Input: part model. Units: mm. Frame: model coordinates. A direction names the side the tool comes from. Give positions to 0.01 mm unless a question says otherwise; leave off trailing zeros. Write each loop counter-clockwise with the first axis right and the second up, starting at its lowest first coordinate (ties: lowest second). Pieces come first, ordered by that corner, then holes.
```python
from build123d import *

# Parameters (mm, degrees)
SKETCH1_R            = 2.9
BOSS_EXTRUDE1_DEPTH  = 7.5
SKETCH2_W            = 1
SKETCH2_H            = 1
CUT_EXTRUDE1_DEPTH   = 7.5
SKETCH8_W            = 1.3
SKETCH8_H            = 7.5
BOSS_EXTRUDE4_DEPTH  = 1
CIRPATTERN3_COUNT    = 8
SKETCH10_W           = 1.3
SKETCH10_H           = 3.5
BOSS_EXTRUDE6_DEPTH  = 1
SKETCH11_W           = 1.3
SKETCH11_H           = 3.5
BOSS_EXTRUDE7_DEPTH  = 1
SKETCH12_W           = 1.3
SKETCH12_H           = 3.5
BOSS_EXTRUDE8_DEPTH  = 1
SKETCH14_W           = 1.3
SKETCH14_H           = 3.5
BOSS_EXTRUDE9_DEPTH  = 1
SKETCH15_W           = 1.3
SKETCH15_H           = 3.5
BOSS_EXTRUDE10_DEPTH = 1
SKETCH16_W           = 1.3
SKETCH16_H           = 3.5
BOSS_EXTRUDE11_DEPTH = 1
SKETCH17_W           = 1.3
SKETCH17_H           = 3.43512081
BOSS_EXTRUDE12_DEPTH = 1
SKETCH18_W           = 1.3
SKETCH18_H           = 3.5
BOSS_EXTRUDE13_DEPTH = 1


with BuildPart() as part:
    # Sketch1 → Boss-Extrude1 (new body)
    with BuildSketch(Plane(origin=(0, 0, 0), x_dir=(1, 0, 0), z_dir=(0, 1, 0))):
        Circle(SKETCH1_R)
    extrude(amount=BOSS_EXTRUDE1_DEPTH)

    # Sketch2 → Cut-Extrude1 (cut)
    with BuildSketch(Plane.XZ):
        with BuildLine():
            Line((0.5, 0.5), (0.5, 2.2))
            ThreePointArc((0.5, 2.2), (0, 2.7), (-0.5, 2.2))
            Line((-0.5, 2.2), (-0.5, 0.5))
            Line((-0.5, 0.5), (0.5, 0.5))
        make_face()
        Rectangle(SKETCH2_W, SKETCH2_H)
        with BuildLine():
            Line((0.5, -2.2), (0.5, -0.5))
            Line((0.5, -0.5), (-0.5, -0.5))
            Line((-0.5, -0.5), (-0.5, -2.2))
            ThreePointArc((-0.5, -2.2), (0, -2.7), (0.5, -2.2))
        make_face()
        with BuildLine():
            Line((2.2, 0.5), (0.5, 0.5))
            Line((0.5, 0.5), (0.5, -0.5))
            Line((0.5, -0.5), (2.2, -0.5))
            ThreePointArc((2.2, -0.5), (2.7, 0), (2.2, 0.5))
        make_face()
        with BuildLine():
            Line((-0.5, -0.5), (-0.5, 0.5))
            Line((-0.5, 0.5), (-2.2, 0.5))
            ThreePointArc((-2.2, 0.5), (-2.7, 0), (-2.2, -0.5))
            Line((-2.2, -0.5), (-0.5, -0.5))
        make_face()
    extrude(amount=-CUT_EXTRUDE1_DEPTH, mode=Mode.SUBTRACT)

    # Sketch8 → Boss-Extrude4 (add)
    with BuildSketch(Plane(origin=(2.8, 0, 0), x_dir=(0, 0, -1), z_dir=(1, 0, 0))):
        with Locations((0.006709133, 3.75)):
            Rectangle(SKETCH8_W, SKETCH8_H)
    boss_extrude4 = extrude(amount=BOSS_EXTRUDE4_DEPTH)

    # CirPattern3: Boss-Extrude4 ×8 about axis
    cirpattern3_axis = Axis((0, 0, 0), (0, 1, 0))
    for i in range(1, CIRPATTERN3_COUNT):
        add(boss_extrude4.rotate(cirpattern3_axis, i * 360 / CIRPATTERN3_COUNT))

    # Sketch10 → Boss-Extrude6 (add)
    with BuildSketch(Plane(origin=(0, 0, -3.8), x_dir=(-1, 0, 0), z_dir=(0, 0, -1))):
        with Locations((0.006709133, 3.75)):
            Rectangle(SKETCH10_W, SKETCH10_H)
    extrude(amount=BOSS_EXTRUDE6_DEPTH)

    # Sketch11 → Boss-Extrude7 (add)
    with BuildSketch(Plane(origin=(-2.687005769, 0, -2.687005769), x_dir=(-0.707106781, 0, 0.707106781), z_dir=(-0.707106781, 0, -0.707106781))):
        with Locations((0.006709133, 3.75)):
            Rectangle(SKETCH11_W, SKETCH11_H)
    extrude(amount=BOSS_EXTRUDE7_DEPTH)

    # Sketch12 → Boss-Extrude8 (add)
    with BuildSketch(Plane.ZY.offset(3.8)):
        with Locations((0.006709133, 3.75)):
            Rectangle(SKETCH12_W, SKETCH12_H)
    extrude(amount=BOSS_EXTRUDE8_DEPTH)

    # Sketch14 → Boss-Extrude9 (add)
    with BuildSketch(Plane(origin=(-2.687005769, 0, 2.687005769), x_dir=(0.707106781, 0, 0.707106781), z_dir=(-0.707106781, 0, 0.707106781))):
        with Locations((0.006709133, 3.75)):
            Rectangle(SKETCH14_W, SKETCH14_H)
    extrude(amount=BOSS_EXTRUDE9_DEPTH)

    # Sketch15 → Boss-Extrude10 (add)
    with BuildSketch(Plane.XY.offset(3.8)):
        with Locations((0.006709133, 3.75)):
            Rectangle(SKETCH15_W, SKETCH15_H)
    extrude(amount=BOSS_EXTRUDE10_DEPTH)

    # Sketch16 → Boss-Extrude11 (add)
    with BuildSketch(Plane(origin=(2.687005769, 0, 2.687005769), x_dir=(0.707106781, 0, -0.707106781), z_dir=(0.707106781, 0, 0.707106781))):
        with Locations((0.006709133, 3.75)):
            Rectangle(SKETCH16_W, SKETCH16_H)
    extrude(amount=BOSS_EXTRUDE11_DEPTH)

    # Sketch17 → Boss-Extrude12 (add)
    with BuildSketch(Plane(origin=(3.8, 0, 0), x_dir=(0, 0, -1), z_dir=(1, 0, 0))):
        with Locations((0.006709133, 3.782439595)):
            Rectangle(SKETCH17_W, SKETCH17_H)
    extrude(amount=BOSS_EXTRUDE12_DEPTH)

    # Sketch18 → Boss-Extrude13 (add)
    with BuildSketch(Plane(origin=(2.687005769, 0, -2.687005769), x_dir=(-0.707106781, 0, -0.707106781), z_dir=(0.707106781, 0, -0.707106781))):
        with Locations((0.006709133, 3.75)):
            Rectangle(SKETCH18_W, SKETCH18_H)
    extrude(amount=BOSS_EXTRUDE13_DEPTH)


solid = part.part
```
Q1. Access query for faces 1 (the flat face through (4, 5.5, 0)), 2 (the flat face through (2.99, 3.7, -2.08)), 3 (the flat face through (2.07, 3.7, -3)), 4 (the flat face through (-2.689, 1.014, 2.685)). Directions: +Z, -Z, +X, -X, +Y, -Y. A direction counts if a zero-diameter tool reaches every point of the face in a straight line with its end or side. Return the directions, or none.
Q2. Mould query, pull axis Z, two halves, no side actions, for faces 5 (the flat face through (-0.5, 4, 1)), 6 (the flat face through (0, 4, -4.8)), 7 (the flat face through (3, 2, 3)), 8 (the flat face through (-2.99, 3.7, 2.08)). Classes: +Z half, -Z half, draft (parallel to the pull), parting line (faces both ways), or undercut.
Q3. Pin query (flat end, axial travel): pin 1 (0.6 mm diameter, centred on y = 4.5, z = -4, fed in from -X); pin 2 (0.8 mm diameter, centred on x = -1.5, y = 2, fed in from -Z); pin 3 (2 mm diameter, centred on x = 3.5, y = 3, fed in from +Z). Return the tip coordinate at first contact, or that it passes through.
Q4. Material intervals for line 1 along X through (y, z) = (4.75, 0); line 2 along Z through (x, y) = (0, 6.25); line 3 along X through (y, z) = (2.25, 3.25), sorted ascending.
Q5. Section A-A, the plane x = 0. Return the cut outline in (y, z).
Q6. Section B-B, the plane z = 0. Return the cut outline in (x, y), then the cut area to 3 significant figures.
Q7. Section D-D, the plane x = -1.25. Return the cut outline in (y, z).
Q8. Section C-C, the plane z = -2. Return the cut outline in (x, y).
Solutions:
1. face 1: +Z, -Z, +X, +Y
1. face 2: +X, +Y, -Y
1. face 3: -Z, +Y, -Y
1. face 4: +Z, -X, -Y
2. face 5: undercut
2. face 6: -Z half
2. face 7: draft
2. face 8: undercut
3. pin 1: stops at x = -3.09
3. pin 2: stops at z = -2.81
3. pin 3: stops at z = 3.85
4. line 1: x = -4.8 to -2.7, 2.7 to 4.8
4. line 2: z = -3.8 to -2.7, 2.7 to 3.8
4. line 3: x = -3.54 to -2.32, -0.64 to 0.66, 2.34 to 3.54
5. outline: (0, -3.8) - (2, -3.8) - (2, -4.8) - (5.5, -4.8) - (5.5, -3.8) - (7.5, -3.8) - (7.5, -2.7) - (0, -2.7) - close; (0, 2.7) - (7.5, 2.7) - (7.5, 3.8) - (5.5, 3.8) - (5.5, 4.8) - (2, 4.8) - (2, 3.8) - (0, 3.8) - close
6. outline: (-4.8, 2) - (-3.8, 2) - (-3.8, 0) - (-2.7, 0) - (-2.7, 7.5) - (-3.8, 7.5) - (-3.8, 5.5) - (-4.8, 5.5) - close; (2.7, 0) - (3.8, 0) - (3.8, 2.06) - (4.8, 2.06) - (4.8, 5.5) - (3.8, 5.5) - (3.8, 7.5) - (2.7, 7.5) - close
6. area: 23.4 mm2
7. outline: (0, -2.62) - (7.5, -2.62) - (7.5, -0.5) - (0, -0.5) - close; (0, 0.5) - (7.5, 0.5) - (7.5, 2.62) - (0, 2.62) - close
8. outline: (-2.93, 0) - (-0.5, 0) - (-0.5, 7.5) - (-2.93, 7.5) - close; (0.5, 0) - (2.91, 0) - (2.91, 7.5) - (0.5, 7.5) - close
